from build123d import *

# Parameters (mm, degrees)
SKETCH1_W                                       = 75
SKETCH1_H                                       = 50
BOSS_EXTRUDE1_DEPTH                             = 5
SKETCH2_W                                       = 75
SKETCH2_H                                       = 59
SKETCH2_W_2                                     = 49
SKETCH2_H_2                                     = 28
BOSS_EXTRUDE2_DEPTH                             = 5
BOSS_EXTRUDE3_DEPTH                             = 5
BOSS_EXTRUDE4_START                             = -75
BOSS_EXTRUDE4_DEPTH                             = 5
CBORE_FOR_M3_SHCS1_D                            = 5.25
CBORE_FOR_M3_SHCS1_DEPTH                        = 5
CBORE_FOR_M3_SHCS1_CBORE_D                      = 6
CBORE_FOR_M3_SHCS1_CBORE_DEPTH                  = 0.5
CBORE_FOR_M3_SHCS1_TIP                          = 1.577259125
CSK_FOR_M3_FLAT_HEAD_MACHINE_SCREW1_D           = 3.4
CSK_FOR_M3_FLAT_HEAD_MACHINE_SCREW1_CSINK_D     = 6.3
CSK_FOR_M3_FLAT_HEAD_MACHINE_SCREW1_CSINK_ANGLE = 90


with BuildPart() as part:
    # Sketch1 → Boss-Extrude1 (new body)
    with BuildSketch(Plane(origin=(0, 0, 0), x_dir=(1, 0, 0), z_dir=(0, 1, 0))):
        Rectangle(SKETCH1_W, SKETCH1_H)
    extrude(amount=BOSS_EXTRUDE1_DEPTH)

    # Sketch2 → Boss-Extrude2 (add)
    with BuildSketch(Plane.XY.offset(25)):
        with Locations((0, 34.5)):
            Rectangle(SKETCH2_W, SKETCH2_H)
        with Locations((0, 32)):
            Rectangle(SKETCH2_W_2, SKETCH2_H_2, mode=Mode.SUBTRACT)
    extrude(amount=-BOSS_EXTRUDE2_DEPTH)

    # Sketch3 → Boss-Extrude3 (add)
    with BuildSketch(Plane(origin=(37.5, 0, 0), x_dir=(0, 0, -1), z_dir=(1, 0, 0))):
        Polygon((-20, 64), (25, 5), (-20, 5), align=None)
    extrude(amount=-BOSS_EXTRUDE3_DEPTH)

    # Sketch3<2> → Boss-Extrude4 (add)
    with BuildSketch(Plane(origin=(37.5, 0, 0), x_dir=(0, 0, -1), z_dir=(1, 0, 0)).offset(BOSS_EXTRUDE4_START)):
        Polygon((-20, 64), (25, 5), (-20, 5), align=None)
    extrude(amount=BOSS_EXTRUDE4_DEPTH)

    # CBORE for M3 SHCS1
    with Locations(Plane.XY.offset(25)):
        with Locations((0, 52), (0, 12)):
            CounterBoreHole(CBORE_FOR_M3_SHCS1_D / 2, CBORE_FOR_M3_SHCS1_CBORE_D / 2, CBORE_FOR_M3_SHCS1_CBORE_DEPTH, depth=CBORE_FOR_M3_SHCS1_DEPTH)
            with Locations((0, 0, -(CBORE_FOR_M3_SHCS1_DEPTH + CBORE_FOR_M3_SHCS1_TIP / 2))):  # 118° drill point
                Cone(0, CBORE_FOR_M3_SHCS1_D / 2, CBORE_FOR_M3_SHCS1_TIP, mode=Mode.SUBTRACT)

    # CSK for M3 Flat Head Machine Screw1 (through all)
    with Locations(Plane(origin=(0, 5, 0), x_dir=(1, 0, 0), z_dir=(0, 1, 0))):
        with Locations((22.5, 15), (0, 0), (-22.5, 15), (-22.5, -15), (22.5, -15)):
            CounterSinkHole(CSK_FOR_M3_FLAT_HEAD_MACHINE_SCREW1_D / 2, CSK_FOR_M3_FLAT_HEAD_MACHINE_SCREW1_CSINK_D / 2, counter_sink_angle=CSK_FOR_M3_FLAT_HEAD_MACHINE_SCREW1_CSINK_ANGLE)


solid = part.part
Could you check a few things on this model? Use its own coordinates, in mm. A direction names the side the tool comes from. Give positions to 0.01 mm unless a question says otherwise; leave off trailing zeros. Write each loop counter-clockwise with the first axis right and the second up, starting at its lowest first coordinate (ties: lowest second). Pieces come first, ordered by that corner, then holes. Notation, with made-up numbers: (71, -24) - (90, -24) arc R25 cw to (90, 14) - close; hole circle Ø10 at (-2, 65.5). An arc over 180 degrees is marked (long way). Use CSV: the item, a comma, the result in double quotes. Start each with the question number.
Item 1: If we mould it in two halves opening along X, with no side actions, what happens to faces 6 (the face through (-35.035, 34.913, -2.185)), 7 (the face through (37.5, 25, 5)), 8 (the face through (-0.391, 54.974, 24.754))? For each: pulls with the +X half, pulls with the -X half, needs draft (parallel to the pull), parting line crosses it, or undercut.
Item 2: If I drill on line 1 along X through (y, z) = (2.05, -15); line 2 along Y through (x, z) = (0, 22.55) (3 decimals); line 3 along X through (y, z) = (36, 5), over which ranges is the centre line in solid material (lowest first)?
Item 3: I want a section at D-D, the plane z = 15. Please give me the cut outline in (x, y).
Item 4: I want a section at C-C, the plane x = 0. Give the number of separate pieces and of enclosed holes in the cut face, then the cut area to 3 significant figures.
Item 5: For faces 1 (the face through (-37.5, 25, 5)), 2 (the face through (24.5, 32, 23)), 3 (the face through (0.37, 1.75, 1.66)), 4 (the face through (2, 50, 24.5)), 5 (the face through (0, 5, -8)), which set-ups out of +Z, -Z, +X, -X, +Y, -Y let a thin tool reach every point of the face, with its end or its side?
Item 6: I'm going to push flat-ended pins straight in: pin 1 (4.5 mm diameter, centred on x = 22.5, z = 15, fed in from +Y); pin 2 (2 mm diameter, centred on x = -12.5, y = 51.5, fed in from -Z); pin 3 (2 mm diameter, centred on x = -8.5, z = -12, fed in from +Y). Where does each tip first touch, or does it pass through?
Item 7: I want a section at B-B, the plane y = 34.5. Please give me the cut outline in (x, z).
Item 8: I want a section at A-A, the plane x = 22.5. Please give me the cut outline in (y, z), then the cut area to 3 significant figures.
Findings:
1,face 6,"needs draft"
1,face 7,"pulls with the +X half"
1,face 8,"undercut"
2,line 1,"x = -37.5 to -24.2, -20.8 to 20.8, 24.2 to 37.5"
2,line 2,"y = 0 to 9.375, 14.625 to 18, 46 to 49.375, 54.625 to 64"
2,line 3,"x = -37.5 to -32.5, 32.5 to 37.5"
3,outline,"(-37.5, 0) - (-24.2, 0) - (-24.2, 3.55) - (-25.65, 5) - (-32.5, 5) - (-32.5, 57.44) - (-37.5, 57.44) - close; (-20.8, 0) - (20.8, 0) - (20.8, 3.55) - (19.35, 5) - (-19.35, 5) - (-20.8, 3.55) - close; (24.2, 0) - (37.5, 0) - (37.5, 57.44) - (32.5, 57.44) - (32.5, 5) - (25.65, 5) - (24.2, 3.55) - close"
4,separate pieces,"5"
4,enclosed holes,"0"
4,area,"333 mm2"
5,face 1,"+Z, -Z, -X, +Y, -Y"
5,face 2,"+Z, -Z"
5,face 3,"+Y, -Y"
5,face 4,"+Z"
5,face 5,"-Z, +Y"
6,pin 1,"stops at y = 4.1"
6,pin 2,"stops at z = 20"
6,pin 3,"stops at y = 5"
7,outline,"(-37.5, -2.5) - (-32.5, -2.5) - (-32.5, 20) - (-24.5, 20) - (-24.5, 25) - (-37.5, 25) - close; (24.5, 20) - (32.5, 20) - (32.5, -2.5) - (37.5, -2.5) - (37.5, 25) - (24.5, 25) - close"
8,outline,"(0, -25) - (5, -25) - (5, -18.15) - (3.55, -16.7) - (0, -16.7) - close; (0, -13.3) - (3.55, -13.3) - (5, -11.85) - (5, 11.85) - (3.55, 13.3) - (0, 13.3) - close; (0, 16.7) - (3.55, 16.7) - (5, 18.15) - (5, 20) - (18, 20) - (18, 25) - (0, 25) - close; (46, 20) - (64, 20) - (64, 25) - (46, 25) - close"
8,area,"367 mm2"
